The listing builds one solid part. Answer for the finished solid, in the listing's coordinates (mm). A direction names the side the tool comes from. Give positions to 0.01 mm unless a question says otherwise; leave off trailing zeros. Write each loop counter-clockwise with the first axis right and the second up, starting at its lowest first coordinate (ties: lowest second). Pieces come first, ordered by that corner, then holes. Notation, with made-up numbers: (81.5, 38) - (110.5, 38) arc R30 cw to (110.5, 71) - close; hole circle Ø3 at (52.25, -19.5). An arc over 180 degrees is marked (long way). Use a Markdown table: item, result. Add a question column.
Autodesk Inventor part; units mm, degrees
ref_plane "YZ Plane" through (0, 0, 0) normal (1, 0, 0) x (0, 1, 0)
ref_plane "XZ Plane" through (0, 0, 0) normal (0, 1, 0) x (-1, 0, 0)
ref_plane "XY Plane" through (0, 0, 0) normal (0, 0, 1) x (1, 0, 0)
sketch "Sketch1" plane through (0, 0, 0) normal (0, 1, 0) x (1, 0, 0)
  line L0 (300, 0) -> (-300, 0)
  line L1 (-300, 0) -> (-300, -600)
  line L2 (-300, -600) -> (300, -600)
  line L3 (300, -600) -> (300, 0)
  point P0 (0, 0)
  point P1 (0, 0)
  dimension "d0" = 600
  dimension "d1" = 600
extrude "Extrusion1" add sketch "Sketch1" along normal blind 850
sketch "Sketch2" plane through (-300, 0, 600) normal (0, 0, 1) x (-1, 0, 0)
  line L0 (-600, 0) -> (-600, -850)
  line L1 (-600, 0) -> (-570, 0)
  line L2 (-570, 0) -> (-570, -120)
  line L3 (-570, -120) -> (-600, -120)
  line L4 (-600, -120) -> (-600, 0)
  point P0 (-300, 0)
  dimension "d4" = 120
  dimension "d7" = 30
extrude "Extrusion2" cut sketch "Sketch2" against normal blind 30
move faces "Move3" translate (450, 0, 0) faces at (300, 323.3333, 190)
move faces "Move4" translate (0, 0, 450) faces at (240, 606.6667, 600)
sketch "Sketch3" plane through (270, 120, 570) normal (0, -1, 0) x (1, 0, 0)
  line L0 (-570, 480) -> (480, 480)
  line L1 (480, 480) -> (30, 480)
  line L2 (30, 480) -> (30, 30)
  line L3 (30, 30) -> (480, 30)
  line L4 (480, 30) -> (480, 480)
  line L5 (-570, 480) -> (-570, -570)
  line L6 (-570, -570) -> (480, -570)
  point P0 (-270, -570)
  point P1 (30, 480)
  dimension "d20" = 600
  dimension "d21" = 600
extrude "Extrusion3" cut sketch "Sketch3" against normal through all
sketch "Sketch4" plane through (0, 850, 0) normal (0, 1, 0) x (1, 0, 0)
  line L0 (-240, -293.3452) -> (-6.6548, -60)
  line L1 (-6.6548, -60) -> (570, -60)
  line L2 (570, -60) -> (570, -540)
  line L3 (570, -540) -> (240, -540)
  line L4 (240, -540) -> (240, -870)
  line L5 (240, -870) -> (-240, -870)
  line L6 (-240, -870) -> (-240, -293.3452)
  line L7 (300, -600) -> (300, -1050) construction
  line L8 (240, -540) -> (300, -600) construction
  line L9 (-300, 0) -> (-300, -1050)
  point P0 (0, 0)
  point P1 (0, -870)
  dimension "d24" = 480
  dimension "d25" = 330
  dimension "d26" = 810
  dimension "d27" = 576.6548
  dimension "d28" = 330
  dimension "d29" = 300
extrude "Extrusion4" cut sketch "Sketch4" against normal blind 260
equation "\"d19\" = d16"
properties part number "Mobile lavandino angolo"
1. The part is cut by section C-C (z = 387.5). Give the vertices of the cut face in (x, y), and give its area (3 significant figures).
2. Consider L1, parallel to Z at x = 125.5, y = 709.5; L2, parallel to X at y = 797, z = 349; L3, parallel to X at y = 749, z = 867.5. Determine where each line is inside the solid, lowest interval first. Write a range as [from, to].
3. The part is cut by section D-D (y = 510.5). Give the vertices of the cut face in (x, z), and give its area (3 significant figures).
4. The part is cut by section B-B (x = 155.5). Give the vertices of the cut face in (y, z), and give its area (3 significant figures).
5. Which of the six approach directions +Z, -Z, +X, -X, +Y, -Y give full straight-line access (tool end or side, diameter ignored) to faces 1 (the flat face through (407, 722, 540)), 2 (the flat face through (300, 480, 828)), 3 (the flat face through (270, 59, 813))?
6. Given P1, Ø1, axis at y = 504.5, z = 895, coming from the +X side; P2, Ø8, axis at x = 638, y = 582.5, coming from the +Z side, each flat-ended and moving along its own axis, determine where each tip first touches the part or whether it passes through.
7. For a pull along Z with two mould halves and no side action, classify faces 4 (the flat face through (750, 419, 304)), 5 (the flat face through (3, 722, 870)), 6 (the flat face through (522, 480, 600)) as released by +Z, released by -Z, zero draft, split by the parting line, or undercut.
8. The part is cut by section A-A (y = 797.5). Give the vertices of the cut face in (x, z).
Check values:
| question | item | result |
|---|---|---|
| 1 | outline | (-300, 0) - (750, 0) - (750, 850) - (570, 850) - (570, 590) - (-240, 590) - (-240, 850) - (-300, 850) - close |
| 1 | area | 682,000 mm2 |
| 2 | L1 | z = [0, 60], [870, 1050] |
| 2 | L2 | x = [-300, -240], [570, 750] |
| 2 | L3 | x = [-300, -240], [240, 300] |
| 3 | outline | (-300, 0) - (750, 0) - (750, 600) - (300, 600) - (300, 1050) - (-300, 1050) - close |
| 3 | area | 900,000 mm2 |
| 4 | outline | (0, 0) - (850, 0) - (850, 60) - (590, 60) - (590, 870) - (850, 870) - (850, 1050) - (0, 1050) - close |
| 4 | area | 682,000 mm2 |
| 5 | face 1 | +Y |
| 5 | face 2 | +Z, +X, +Y, -Y |
| 5 | face 3 | +Z, +X, -Y |
| 6 | P1 | stops at x = 300 |
| 6 | P2 | stops at z = 600 |
| 7 | face 4 | zero draft |
| 7 | face 5 | undercut |
| 7 | face 6 | released by +Z |
| 8 | outline | (-300, 0) - (750, 0) - (750, 600) - (300, 600) - (300, 1050) - (-300, 1050) - close; hole (-240, 293.35) - (-6.65, 60) - (570, 60) - (570, 540) - (240, 540) - (240, 870) - (-240, 870) - close |
